Part print with two shaded views. Sizes in mm from the minimum x, y, z corner. Round coordinates to 2 decimals unless told otherwise and drop trailing zeros. Write each loop counter-clockwise with the first axis right and the second up, starting at its lowest first coordinate (ties: lowest second). Pieces come first, ordered by that corner, then holes. Notation, with made-up numbers: M 81.25,-2.75 L 111.25,-2.75 A19 ccw 111.25,16.25 Z; hole C 39,55.25 d8. An arc over 180 degrees is marked long. One line per question, with ' | ' between items. Start each with the question number.
1) Saw through at D-D (y = 141). List the corners of the cut face in (x, z) (1 decimal).
2) Saw through at C-C (z = 109.5). List the corners of the cut face in (x, y) (1 decimal).
3) Wall check: probe 1 along X at (y, z) = (92.5, 25.5); probe 2 along X at (y, z) = (326, 186) (1 decimal); probe 3 along Y at (x, z) = (869, 219) (1 decimal). Give the ranges that are in metal, low to high. Write a range as [from, to].
4) Saw through at A-A (y = 559). List the corners of the cut face in (x, z) (1 decimal).
5) Drop flat-ended pins along their axis: pin 1 Ø10 at (y, z) = (232, 350) entering from +X; pin 2 Ø3 at (y, z) = (434.5, 369) entering from +X (1 decimal). Give the stop position or say it passes through.
6) Saw through at B-B (x = 239.5). List the corners of the cut face in (y, z) (1 decimal).
7) Mould opens along X. For the marked faces 1, 2, 3 and 4 say: pulls with the +X half, pulls with the -X half, needs draft (parallel to the pull), parting line crosses it, or undercut.
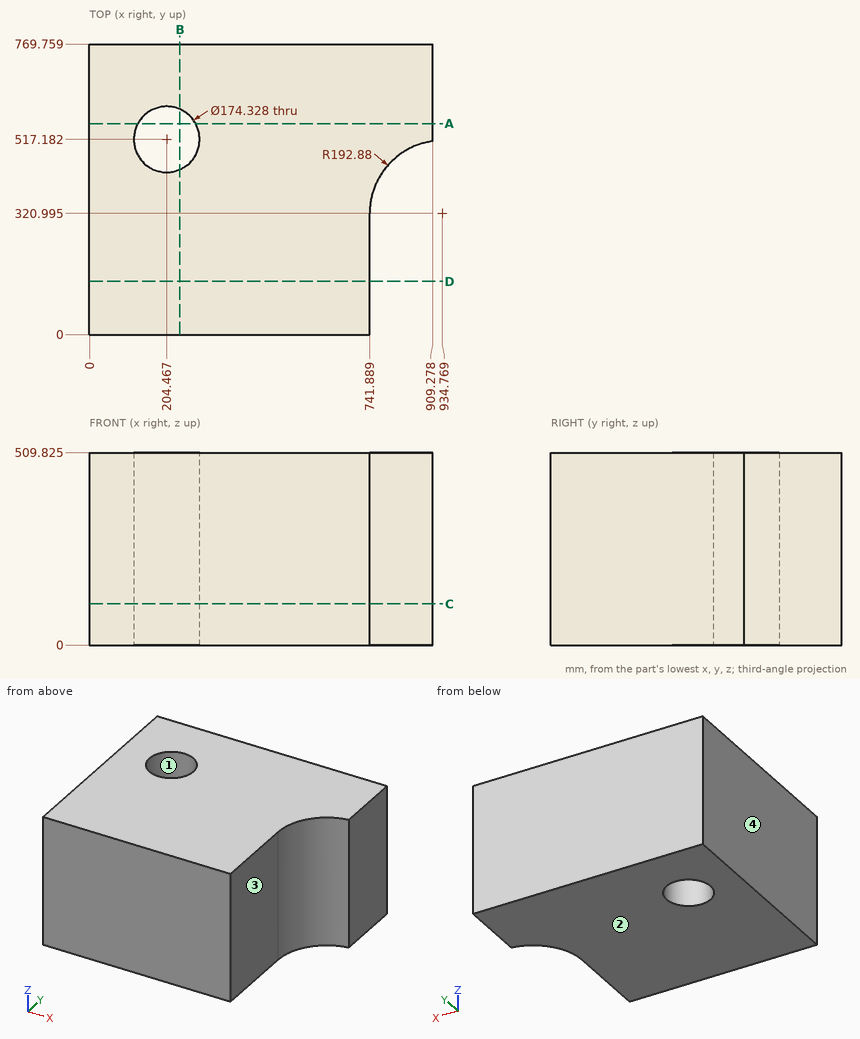
Answer key:
1) outline: M 0,0 L 741.9,0 L 741.9,509.8 L 0,509.8 Z
2) outline: M 0,0 L 741.9,0 L 741.9,321 A192.9 cw 909.3,512.2 L 909.3,769.8 L 0,769.8 Z; hole C 204.5,517.2 d174.3
3) probe 1: x = [0, 741.89] | probe 2: x = [0, 742] | probe 3: y = [502.3, 769.8]
4) outline: M 0,0 L 128,0 L 128,509.8 L 0,509.8 Z; M 280.9,0 L 909.3,0 L 909.3,509.8 L 280.9,509.8 Z
5) pin 1: stops at x = 741.89 | pin 2: stops at x = 779.9
6) outline: M 0,0 L 437.4,0 L 437.4,509.8 L 0,509.8 Z; M 597,0 L 769.8,0 L 769.8,509.8 L 597,509.8 Z
7) face 1: undercut | face 2: needs draft | face 3: pulls with the +X half | face 4: pulls with the -X half
